from build123d import *

# Parameters (mm, degrees)
F0_R     = 27.432
F1_DEPTH = 10.16


with BuildPart() as f1:
    # F0 (on Front) → F1 (new body)
    with BuildSketch(Plane.XZ):
        with BuildLine():
            ThreePointArc((0, -38.4786100226), (11.1592316368, -65.4193783858), (38.1, -76.5786100226))
            Line((38.1, -76.5786100226), (106.68, -76.5786100226))
            ThreePointArc((106.68, -76.5786100226), (133.6207683632, -65.4193783858), (144.78, -38.4786100226))
            Line((144.78, -38.4786100226), (144.78, 174.1193899774))
            ThreePointArc((144.78, 174.1193899774), (133.6207683632, 201.0601583406), (106.68, 212.2193899774))
            Line((106.68, 212.2193899774), (38.1, 212.2193899774))
            ThreePointArc((38.1, 212.2193899774), (11.1592316368, 201.0601583406), (0, 174.1193899774))
            Line((0, 174.1193899774), (0, -38.4786100226))
        make_face()
        Polygon((22.1777712578, -33.1991309873), (22.1777712578, -56.8850969951), (25.7456152258, -57.4299074334), (25.7456152258, -58.9646783023), (12.065558, -58.9646783023), (12.065558, -57.4299074334), (15.6334019681, -56.8850969951), (15.6334019681, -33.1991309873), (12.065558, -32.6343884598), (12.065558, -31.11954968), (25.7456152258, -31.11954968), (25.7456152258, -32.6343884598), align=None, mode=Mode.SUBTRACT)
        with BuildLine():
            Line((21.845569771, -10.0646194476), (6.4380648139, -10.0646194476))
            Line((6.4380648139, -10.0646194476), (6.4380648139, -8.5497806678))
            Line((6.4380648139, -8.5497806678), (10.8563445881, -7.9850381403))
            Line((10.8563445881, -7.9850381403), (10.8563445881, 15.5746913025))
            Line((10.8563445881, 15.5746913025), (9.7999438602, 15.5746913025))
            add(Edge.make_bspline(
                [(9.7999438602, 15.5746913025), (5.0428185694, 15.5746913025), (3.116049946, 15.1627614589)],
                knots=[0, 0, 0, 1, 1, 1], degree=2))
            Line((3.116049946, 15.1627614589), (2.5513074185, 9.9937063245))
            Line((2.5513074185, 9.9937063245), (0.6644029736, 9.9937063245))
            Line((0.6644029736, 9.9937063245), (0.6644029736, 17.7805091747))
            Line((0.6644029736, 17.7805091747), (27.7188920573, 17.7805091747))
            Line((27.7188920573, 17.7805091747), (27.7188920573, 9.9937063245))
            Line((27.7188920573, 9.9937063245), (25.8054114935, 9.9937063245))
            Line((25.8054114935, 9.9937063245), (25.2473129957, 15.1627614589))
            add(Edge.make_bspline(
                [(25.2473129957, 15.1627614589), (23.5265092941, 15.5348271241), (18.4371825166, 15.5348271241)],
                knots=[0, 0, 0, 1, 1, 1], degree=2))
            Line((18.4371825166, 15.5348271241), (17.420645967, 15.5348271241))
            Line((17.420645967, 15.5348271241), (17.420645967, -7.9850381403))
            Line((17.420645967, -7.9850381403), (21.845569771, -8.5497806678))
            Line((21.845569771, -8.5497806678), (21.845569771, -10.0646194476))
        make_face(mode=Mode.SUBTRACT)
        Polygon((5.3152237886, 40.9150207144), (8.8897117864, 40.3502781869), (8.8897117864, 38.8354394072), (0.4185738733, 38.8354394072), (0.4185738733, 40.3502781869), (2.4915111509, 40.9150207144), (12.3977594868, 66.9064650405), (18.4172504274, 66.9064650405), (28.2769905551, 40.9150207144), (30.3964360408, 40.3502781869), (30.3964360408, 38.8354394072), (17.998676554, 38.8354394072), (17.998676554, 40.3502781869), (21.2210309758, 40.9150207144), (18.5634190815, 48.1171489479), (7.8665312071, 48.1171489479), align=None, mode=Mode.SUBTRACT)
        with BuildLine():
            Line((14.5969333293, 98.6582831474), (10.8563445881, 98.6582831474))
            Line((10.8563445881, 98.6582831474), (10.8563445881, 89.8150795692))
            Line((10.8563445881, 89.8150795692), (15.4872333139, 89.2503370416))
            Line((15.4872333139, 89.2503370416), (15.4872333139, 87.7354982619))
            Line((15.4872333139, 87.7354982619), (0.9966044604, 87.7354982619))
            Line((0.9966044604, 87.7354982619), (0.9966044604, 89.2503370416))
            Line((0.9966044604, 89.2503370416), (4.298687239, 89.8150795692))
            Line((4.298687239, 89.8150795692), (4.298687239, 113.5209776661))
            Line((4.298687239, 113.5209776661), (0.7241992412, 114.0657881045))
            Line((0.7241992412, 114.0657881045), (0.7241992412, 115.5806268842))
            Line((0.7241992412, 115.5806268842), (12.995722163, 115.5806268842))
            add(Edge.make_bspline(
                [(12.995722163, 115.5806268842), (18.9155526575, 115.5806268842), (21.8422477561, 113.5973840081)],
                knots=[0, 0, 0, 1, 1, 1], degree=2))
            add(Edge.make_bspline(
                [(21.8422477561, 113.5973840081), (24.7689428547, 111.614141132), (24.7689428547, 107.3752501606)],
                knots=[0, 0, 0, 1, 1, 1], degree=2))
            add(Edge.make_bspline(
                [(24.7689428547, 107.3752501606), (24.7689428547, 98.6582831474), (14.5969333293, 98.6582831474)],
                knots=[0, 0, 0, 1, 1, 1], degree=2))
        make_face(mode=Mode.SUBTRACT)
        with BuildLine():
            Line((0.7241992412, 136.6355571166), (0.7241992412, 138.1503958964))
            Line((0.7241992412, 138.1503958964), (4.298687239, 138.7151384239))
            Line((4.298687239, 138.7151384239), (4.298687239, 162.4210365209))
            Line((4.298687239, 162.4210365209), (0.7241992412, 162.9658469592))
            Line((0.7241992412, 162.9658469592), (0.7241992412, 164.4806857389))
            Line((0.7241992412, 164.4806857389), (24.4367413679, 164.4806857389))
            Line((24.4367413679, 164.4806857389), (24.4367413679, 157.3981500407))
            Line((24.4367413679, 157.3981500407), (22.549836923, 157.3981500407))
            Line((22.549836923, 157.3981500407), (21.8854339494, 161.9028022015))
            add(Edge.make_bspline(
                [(21.8854339494, 161.9028022015), (19.5600235419, 162.1951395099), (15.1550318271, 162.1951395099)],
                knots=[0, 0, 0, 1, 1, 1], degree=2))
            Line((15.1550318271, 162.1951395099), (10.8364124989, 162.1951395099))
            Line((10.8364124989, 162.1951395099), (10.8364124989, 151.9766217764))
            Line((10.8364124989, 151.9766217764), (18.124913119, 151.9766217764))
            Line((18.124913119, 151.9766217764), (18.7693840033, 155.052807544))
            Line((18.7693840033, 155.052807544), (20.6164242699, 155.052807544))
            Line((20.6164242699, 155.052807544), (20.6164242699, 146.4952972444))
            Line((20.6164242699, 146.4952972444), (18.7693840033, 146.4952972444))
            Line((18.7693840033, 146.4952972444), (18.124913119, 149.6512113689))
            Line((18.124913119, 149.6512113689), (10.8364124989, 149.6512113689))
            Line((10.8364124989, 149.6512113689), (10.8364124989, 138.9211033457))
            Line((10.8364124989, 138.9211033457), (16.0918400199, 138.9211033457))
            add(Edge.make_bspline(
                [(16.0918400199, 138.9211033457), (21.4469279868, 138.9211033457), (23.1079354208, 139.2533048325)],
                knots=[0, 0, 0, 1, 1, 1], degree=2))
            Line((23.1079354208, 139.2533048325), (24.2905727137, 144.4024278777))
            Line((24.2905727137, 144.4024278777), (26.1841211884, 144.4024278777))
            Line((26.1841211884, 144.4024278777), (25.7854794042, 136.6355571166))
            Line((25.7854794042, 136.6355571166), (0.7241992412, 136.6355571166))
        make_face(mode=Mode.SUBTRACT)
        with Locations((74.0844953617, 167.8276180772)):
            Circle(F0_R, mode=Mode.SUBTRACT)
    extrude(amount=F1_DEPTH)


solid = f1.part
Can you work these out from the model? Positions are in its coordinate system, mm. A direction names the side the tool comes from. Coordinates: 2 decimals unless noted, no trailing zeros. Order: outer loops, then holes, each group sorted by start corner. A loop starts at its lowest first (then second) coordinate and runs counter-clockwise, first axis right, second up. Notation, with made-up numbers: M -1.75,-35.5 L 24.25,-35.5 A15 cw 24.25,-24.5 Z; hole C 2.5,68 d4. An arc over 180 degrees is marked long. Answer as CSV lines item,"result".
(1) I'm going to push flat-ended pins straight in: pin 1 (3 mm diameter, centred on x = 5, y = -6, fed in from -Z); pin 2 (1 mm diameter, centred on x = 26.5, y = -4, fed in from +Z); pin 3 (3 mm diameter, centred on y = -7, z = 159.5, fed in from -X); pin 4 (1.2 mm diameter, centred on y = -3, z = -58.5, fed in from +X). Where does each tip first touch, or does it pass through?
Geometry check:
pin 1,"z = -59.76"
pin 2,"z = 210.57"
pin 3,"x = 0"
pin 4,"x = 139.46"
(2) If we mould it in two halves opening along Z, with no side actions, what happens to faces 1 (the flat face through (0.664, -5, 14)), 2 (the cylindrical face through (133.92, -5.01, 200.76)), 3 (the flat face through (72, -5, -76.579))? For each: released by +Z, released by -Z, zero draft, split by the parting line, or undercut.
Geometry check:
face 1,"undercut"
face 2,"released by +Z"
face 3,"released by -Z"
(3) Please list where these lines run through material, in increasing order: L1, parallel to Z at x = 50, y = -2; L2, parallel to X at y = -6.5, z = -45; L3, parallel to Z at x = 107, y = -8.5.
Geometry check:
L1,"-76.58 to 154.7, 180.96 to 212.22"
L2,"0.56 to 15.63, 22.18 to 144.22"
L3,"-76.58 to 212.22"
(4) Suppose I cut it at C-C on y = -2.75. Count the separate pieces of the cut face and the enclosed holes in it, plus the area to 3 significant figures.
Geometry check:
separate pieces,"1"
enclosed holes,"6"
area,"36,600 mm^2"
(5) Suppose I cut it at B-B on z = 178. Please give me the cut outline in (x, y).
Geometry check:
outline,"M 0.2,-10.16 L 48.61,-10.16 L 48.61,0 L 0.2,0 Z; M 99.56,-10.16 L 144.58,-10.16 L 144.58,0 L 99.56,0 Z"
(6) On a 3-axis mill with a long thin cutter (end or side, diameter ignored), from which of +Z, -Z, +X, -X, +Y, -Y can I reach the whole of each face in a straight line? I mean faces 4 (the flat face through (4.299, -5, 150)), 5 (the flat face through (71, 0, 70)). Say none if no direction works.
Geometry check:
face 4,"+Y, -Y"
face 5,"+Z, -Z, +X, -X, +Y"
(7) Suppose I cut it at A-A on x = 72. Please give me the cut outline in (y, z).
Geometry check:
outline,"M -10.16,-76.58 L 0,-76.58 L 0,140.47 L -10.16,140.47 Z; M -10.16,195.18 L 0,195.18 L 0,212.22 L -10.16,212.22 Z"
